Can you work these out from the model? Positions are in its coordinate system, mm. A direction names the side the tool comes from. Coordinates: 2 decimals unless noted, no trailing zeros. Loops run counter-clockwise (first coordinate to the right, second up) from the corner with the lowest first, then second, coordinate; pieces in that order, holes last. Notation, with made-up numbers: (36.25, 57.5) -> (95.25, 57.5) arc R34 ccw to (95.25, 89.5) -> close; hole circle Ø3 at (-26.75, 33). An arc over 180 degrees is marked (long way). Use one line per item in the form item = value. Start each with the question number.
(1) Thinking about a two-plate mould opening in Z: for faces 3 (the cylindrical face through (-0.86, -2.461, 3.874)), 4 (the flat face through (-3, 4, 2)), 5 (the cylindrical face through (-3.86, -2.35, -5.04)), which applies, released by +Z, released by -Z, zero draft, split by the parting line, or undercut?
(2) I need wall thicknesses on line 1 (X direction, y = 2.5, z = 0); line 2 (Z direction, x = 3, y = -2.5); line 3 (X direction, y = -1.75, z = 0.5). Which ranges of each line are inside material? Lowest first, please. Write a range as [from, to].
(3) I'm going to push flat-ended pins straight in: pin 1 (1.5 mm diameter, centred on y = 2, z = -2.5, fed in from -X); pin 2 (1.5 mm diameter, centred on x = 4.5, y = -3, fed in from -Z); pin 3 (2 mm diameter, centred on y = 2.5, z = -5, fed in from -X). Where does each tip first touch, or does it pass through?
(4) Imagine slicing it at C-C (y = -2.75). List the corners of the cut face in (x, z) for me.
(5) Imagine slicing it at B-B (y = 0.75). List the corners of the cut face in (x, z) for me.
(6) Imagine slicing it at A-A (y = 2). List the corners of the cut face in (x, z) for me.
(7) On a 3-axis mill with a long thin cutter (end or side, diameter ignored), from which of +Z, -Z, +X, -X, +Y, -Y can I reach the whole of each face in a straight line? I mean faces 1 (the cylindrical face through (0.9, 2.48, 2.86)), 2 (the conical face through (0, 0, 0)). Say none if no direction works.
```python
from build123d import *

# Parameters (mm, degrees)
SKETCH1_R                                = 5
SKETCH1_R_2                              = 3
BOSS_EXTRUDE1_DEPTH                      = 1
SKETCH1_3_R                              = 5
SKETCH1_3_R_2                            = 3
BOSS_EXTRUDE2_DEPTH                      = 4
CHAMFER1_SIZE                            = 0.25
SKETCH5_R                                = 6.35
BOSS_EXTRUDE4_DEPTH                      = 4.7625
F_5_16_0_3125_DIAMETER_HOLE1_D           = 7.9375
F_5_16_0_3125_DIAMETER_HOLE1_DEPTH       = 4.415279367
F_5_16_0_3125_DIAMETER_HOLE1_CSINK_D     = 8.1915
F_5_16_0_3125_DIAMETER_HOLE1_CSINK_ANGLE = 90
F_5_16_0_3125_DIAMETER_HOLE1_TIP         = 0.347220633
CHAMFER2_SIZE                            = 0.25
CHAMFER3_SIZE                            = 0.5


with BuildPart() as part:
    # Sketch1 → Boss-Extrude1 (new body)
    with BuildSketch(Plane(origin=(0, 0, 0), x_dir=(1, 0, 0), z_dir=(0, 1, 0))):
        with Locations(Location((0, 0, 0), (0, 0, 270))):
            Circle(SKETCH1_R)
        Circle(SKETCH1_R_2, mode=Mode.SUBTRACT)
        Circle(SKETCH1_R_2)
    extrude(amount=BOSS_EXTRUDE1_DEPTH)

    # Sketch1_3 → Boss-Extrude2 (add)
    with BuildSketch(Plane(origin=(0, 0, 0), x_dir=(1, 0, 0), z_dir=(0, 1, 0))):
        with Locations(Location((0, 0, 0), (0, 0, 270))):
            Circle(SKETCH1_3_R)
        with Locations(Location((0, 0, 0), (0, 0, 270))):
            Circle(SKETCH1_3_R_2, mode=Mode.SUBTRACT)
    extrude(amount=BOSS_EXTRUDE2_DEPTH)

    # Chamfer1
    chamfer1_edges = [part.edges().sort_by_distance(p)[0] for p in [
        (0, 1, -3),
        (0, 4, -5),
        (0, 4, -3),
    ]]
    chamfer(chamfer1_edges, length=CHAMFER1_SIZE)

    # Sketch5 → Boss-Extrude4 (add)
    with BuildSketch(Plane(origin=(0, 0, 0), x_dir=(1, 0, 0), z_dir=(0, 1, 0))):
        with Locations(Location((0, 0, 0), (0, 0, 270))):
            Circle(SKETCH5_R)
    extrude(amount=-BOSS_EXTRUDE4_DEPTH)

    # 5_16 _0.3125_ Diameter Hole1
    with Locations(Plane(origin=(0, -4.7625, 0), x_dir=(-1, 0, 0), z_dir=(0, -1, 0))):
        with Locations((0, 0)):
            CounterSinkHole(F_5_16_0_3125_DIAMETER_HOLE1_D / 2, F_5_16_0_3125_DIAMETER_HOLE1_CSINK_D / 2, depth=F_5_16_0_3125_DIAMETER_HOLE1_DEPTH, counter_sink_angle=F_5_16_0_3125_DIAMETER_HOLE1_CSINK_ANGLE)
            with Locations((0, 0, -(F_5_16_0_3125_DIAMETER_HOLE1_DEPTH + F_5_16_0_3125_DIAMETER_HOLE1_TIP / 2))):  # 170° drill point
                Cone(0, F_5_16_0_3125_DIAMETER_HOLE1_D / 2, F_5_16_0_3125_DIAMETER_HOLE1_TIP, mode=Mode.SUBTRACT)

    # Chamfer2
    chamfer2_edges = [part.edges().sort_by_distance(p)[0] for p in [
        (0, -4.7625, -6.35),
        (0, 0, -6.35),
    ]]
    chamfer(chamfer2_edges, length=CHAMFER2_SIZE)

    # Chamfer3
    chamfer3_edges = [part.edges().sort_by_distance(p)[0] for p in [
        (0, 0, -5),
    ]]
    chamfer(chamfer3_edges, length=CHAMFER3_SIZE)


solid = part.part
```
Worked out:
q1.face_3 = undercut
q1.face_4 = zero draft
q1.face_5 = split by the parting line
q2.line_1 = [-5, -3], [3, 5]
q2.line_2 = [-5.6, -2.6], [2.6, 5.6]
q2.line_3 = [-6.33, -3.94], [3.94, 6.33]
q3.pin_1 = -4.68
q3.pin_2 = -5.12
q3.pin_3 = -3
q4.outline = circle Ø12.7 at (0, 0); hole circle Ø7.94 at (0, 0)
q5.outline = circle Ø10 at (0, 0)
q6.outline = circle Ø10 at (0, 0); hole circle Ø6 at (0, 0)
q7.face_1 = +Y
q7.face_2 = -Y
